Geometry: final body of the model. Coordinates: model frame, mm. Face numbers are marked on the shaded views. A direction names the side the tool comes from. Round coordinates to 2 decimals unless told otherwise and drop trailing zeros. Write each loop counter-clockwise with the first axis right and the second up, starting at its lowest first coordinate (ties: lowest second). Pieces come first, ordered by that corner, then holes. Notation, with made-up numbers: (-18, -21.75) -> (12, -21.75) arc R15 ccw to (12, -6.75) -> close; hole circle Ø5 at (-3, -8.5). An arc over 180 degrees is marked (long way). Use one line per item in the form item = value. Start each with the question number.
1. Cut plane B-B, the plane y = -0.3. State how many separate pieces and enclosed holes the cut face has, plus the area to 3 significant figures.
2. Pin query (flat end, axial travel): pin 1 Ø12 at (x, z) = (18.5, 4.5) entering from -Y; pin 2 Ø2 at (x, z) = (-12.5, -16.65) entering from -Y; pin 3 Ø2 at (x, z) = (2, 7) entering from +Y; pin 4 Ø3.5 at (x, z) = (12.5, -16.65) entering from -Y. Return the tip coordinate at first contact, or that it passes through.
3. Reachability of the marked faces 1 and 2 from +Z, -Z, +X, -X, +Y, -Y: full face, straight path, thin tool, end or side. Return the list, or none.
4. Cut plane C-C, the plane z = 6.5. Return the cut outline in (x, y).
5. Line query: L1, parallel to Z at x = 12.5, y = 0.6; L2, parallel to X at y = -0.05, z = -2.5; L3, parallel to X at y = -0.6, z = -16. Output: solid intervals per line, ascending.
6. Cut plane A-A, the plane x = -12.5. Return the cut outline in (y, z).
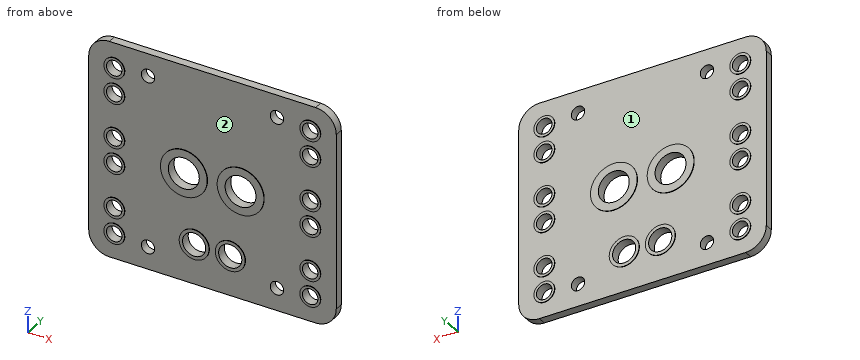
```python
from build123d import *

# Parameters (mm, degrees)
SALIENTE_EXTRUIR1_DEPTH    = 0.8
CROQUIS2_R                 = 1.3
CORTAR_EXTRUIR1_DEPTH      = 1
CORTAR_EXTRUIR1_DEPTH_BACK = 2.6
CROQUIS3_R                 = 3
CORTAR_EXTRUIR2_DEPTH      = 2.6
CROQUIS5_R                 = 4.533685243
CROQUIS5_R_2               = 3
SALIENTE_EXTRUIR2_DEPTH    = 0.9
CROQUIS6_R                 = 2.25
CROQUIS6_R_2               = 1.5
CORTAR_EXTRUIR3_DEPTH      = 2.7
CROQUIS7_R                 = 2
CROQUIS7_R_2               = 1.5
CROQUIS7_R_3               = 2.894896359
CROQUIS7_R_4               = 2.25
SALIENTE_EXTRUIR3_DEPTH    = 0.9


with BuildPart() as part:
    # Croquis1 → Saliente-Extruir1 (new body, symmetric)
    with BuildSketch(Plane(origin=(0, 0, 0), x_dir=(1, 0, 0), z_dir=(0, 1, 0))):
        with BuildLine():
            Line((-20, 21), (20, 21))
            ThreePointArc((20, 21), (22.828427125, 19.828427125), (24, 17))
            Line((24, 17), (24, -17))
            ThreePointArc((24, -17), (22.828427125, -19.828427125), (20, -21))
            Line((20, -21), (-20, -21))
            ThreePointArc((-20, -21), (-22.828427125, -19.828427125), (-24, -17))
            Line((-24, -17), (-24, 17))
            ThreePointArc((-24, 17), (-22.828427125, 19.828427125), (-20, 21))
        make_face()
    extrude(amount=SALIENTE_EXTRUIR1_DEPTH, both=True)

    # Croquis2 → Cortar-Extruir1 (cut, two sides)
    with BuildSketch(Plane(origin=(0, 0.8, 0), x_dir=(1, 0, 0), z_dir=(0, 1, 0))) as cortar_extruir1_sk:
        with Locations((-12.5, 16.65)):
            Circle(CROQUIS2_R)
        with Locations((12.5, 16.65)):
            Circle(CROQUIS2_R)
        with Locations((12.5, -16.65)):
            Circle(CROQUIS2_R)
        with Locations((-12.5, -16.65)):
            Circle(CROQUIS2_R)
    extrude(amount=CORTAR_EXTRUIR1_DEPTH, mode=Mode.SUBTRACT)
    extrude(cortar_extruir1_sk.sketch, amount=-CORTAR_EXTRUIR1_DEPTH_BACK, mode=Mode.SUBTRACT)

    # Croquis3 → Cortar-Extruir2 (cut, through all)
    with BuildSketch(Plane(origin=(0, 0.8, 0), x_dir=(1, 0, 0), z_dir=(0, 1, 0))):
        with Locations((-5.5, 0)):
            Circle(CROQUIS3_R)
        with Locations((5.5, 0)):
            Circle(CROQUIS3_R)
    extrude(amount=-CORTAR_EXTRUIR2_DEPTH, mode=Mode.SUBTRACT)

    # Croquis5 → Saliente-Extruir2 (add, symmetric)
    with BuildSketch(Plane(origin=(0, 0, 0), x_dir=(1, 0, 0), z_dir=(0, 1, 0))):
        with Locations((-5.5, 0)):
            Circle(CROQUIS5_R)
        with Locations((-5.5, 0)):
            Circle(CROQUIS5_R_2, mode=Mode.SUBTRACT)
        with Locations((5.5, 0)):
            Circle(CROQUIS5_R)
        with Locations((5.5, 0)):
            Circle(CROQUIS5_R_2, mode=Mode.SUBTRACT)
    extrude(amount=SALIENTE_EXTRUIR2_DEPTH, both=True)

    # Croquis6 → Cortar-Extruir3 (cut, through all)
    with BuildSketch(Plane(origin=(0, 0.8, 0), x_dir=(1, 0, 0), z_dir=(0, 1, 0))):
        with Locations((-3.5, 13.25)):
            Circle(CROQUIS6_R)
        with Locations((3.5, 13.25)):
            Circle(CROQUIS6_R)
        with Locations((-19, 2.5)):
            Circle(CROQUIS6_R_2)
        with Locations((-19, -2.5)):
            Circle(CROQUIS6_R_2)
        with Locations((-19, 11.14)):
            Circle(CROQUIS6_R_2)
        with Locations((-19, 16.14)):
            Circle(CROQUIS6_R_2)
        with Locations((-19, -11.14)):
            Circle(CROQUIS6_R_2)
        with Locations((-19, -16.14)):
            Circle(CROQUIS6_R_2)
        with Locations((19, -16.14)):
            Circle(CROQUIS6_R_2)
        with Locations((19, -11.14)):
            Circle(CROQUIS6_R_2)
        with Locations((19, 16.14)):
            Circle(CROQUIS6_R_2)
        with Locations((19, 11.14)):
            Circle(CROQUIS6_R_2)
        with Locations((19, -2.5)):
            Circle(CROQUIS6_R_2)
        with Locations((19, 2.5)):
            Circle(CROQUIS6_R_2)
    extrude(amount=-CORTAR_EXTRUIR3_DEPTH, mode=Mode.SUBTRACT)

    # Croquis7 → Saliente-Extruir3 (add, symmetric)
    with BuildSketch(Plane(origin=(0, 0, 0), x_dir=(1, 0, 0), z_dir=(0, 1, 0))):
        with Locations((-19, 16.14)):
            Circle(CROQUIS7_R)
        with Locations((-19, 16.14)):
            Circle(CROQUIS7_R_2, mode=Mode.SUBTRACT)
        with Locations((-19, 11.14)):
            Circle(CROQUIS7_R)
        with Locations((-19, 11.14)):
            Circle(CROQUIS7_R_2, mode=Mode.SUBTRACT)
        with Locations((-19, 2.5)):
            Circle(CROQUIS7_R)
        with Locations((-19, 2.5)):
            Circle(CROQUIS7_R_2, mode=Mode.SUBTRACT)
        with Locations((-19, -2.5)):
            Circle(CROQUIS7_R)
        with Locations((-19, -2.5)):
            Circle(CROQUIS7_R_2, mode=Mode.SUBTRACT)
        with Locations((-19, -16.14)):
            Circle(CROQUIS7_R)
        with Locations((-19, -16.14)):
            Circle(CROQUIS7_R_2, mode=Mode.SUBTRACT)
        with Locations((-19, -11.14)):
            Circle(CROQUIS7_R)
        with Locations((-19, -11.14)):
            Circle(CROQUIS7_R_2, mode=Mode.SUBTRACT)
        with Locations((-3.5, 13.25)):
            Circle(CROQUIS7_R_3)
        with Locations((-3.5, 13.25)):
            Circle(CROQUIS7_R_4, mode=Mode.SUBTRACT)
        with Locations((3.5, 13.25)):
            Circle(CROQUIS7_R_3)
        with Locations((3.5, 13.25)):
            Circle(CROQUIS7_R_4, mode=Mode.SUBTRACT)
        with Locations((19, -11.14)):
            Circle(CROQUIS7_R)
        with Locations((19, -11.14)):
            Circle(CROQUIS7_R_2, mode=Mode.SUBTRACT)
        with Locations((19, -16.14)):
            Circle(CROQUIS7_R)
        with Locations((19, -16.14)):
            Circle(CROQUIS7_R_2, mode=Mode.SUBTRACT)
        with Locations((19, -2.5)):
            Circle(CROQUIS7_R)
        with Locations((19, -2.5)):
            Circle(CROQUIS7_R_2, mode=Mode.SUBTRACT)
        with Locations((19, 2.5)):
            Circle(CROQUIS7_R)
        with Locations((19, 2.5)):
            Circle(CROQUIS7_R_2, mode=Mode.SUBTRACT)
        with Locations((19, 11.14)):
            Circle(CROQUIS7_R)
        with Locations((19, 11.14)):
            Circle(CROQUIS7_R_2, mode=Mode.SUBTRACT)
        with Locations((19, 16.14)):
            Circle(CROQUIS7_R)
        with Locations((19, 16.14)):
            Circle(CROQUIS7_R_2, mode=Mode.SUBTRACT)
    extrude(amount=SALIENTE_EXTRUIR3_DEPTH, both=True)


solid = part.part
```
Outcome:
q1.separate_pieces = 1
q1.enclosed_holes = 20
q1.area = 1,810 mm^2
q2.pin_1 = -0.9
q2.pin_2 = through
q2.pin_3 = 0.8
q2.pin_4 = -0.8
q3.face_1 = +Y
q3.face_2 = -Y
q4.outline = (-24, -0.8) -> (24, -0.8) -> (24, 0.8) -> (-24, 0.8) -> close
q5.L1 = -21 to -17.95, -15.35 to 15.35, 17.95 to 21
q5.L2 = -24 to -20.5, -17.5 to -7.16, -3.84 to 3.84, 7.16 to 17.5, 20.5 to 24
q5.L3 = -24 to -20.49, -17.51 to -13.63, -11.37 to 11.37, 13.63 to 17.51, 20.49 to 24
q6.outline = (-0.8, -21) -> (0.8, -21) -> (0.8, -17.95) -> (-0.8, -17.95) -> close; (-0.8, -15.35) -> (0.8, -15.35) -> (0.8, 15.35) -> (-0.8, 15.35) -> close; (-0.8, 17.95) -> (0.8, 17.95) -> (0.8, 21) -> (-0.8, 21) -> close
